```python
from build123d import *

# Parameters (mm, degrees)
SKETCH_1_R          = 26
SKETCH_1_R_2        = 24
EXTRUDE_1_DEPTH     = 12.6
EXTRUDE_START       = -2
SKETCH_2_R          = 28
SKETCH_2_R_2        = 26
EXTRUDE_2_DEPTH     = 2
SKETCH_3_R          = 26
EXTRUDE_3_DEPTH     = 2
SKETCH_4_R          = 26
SKETCH_4_R_2        = 22
EXTRUDE_4_DEPTH     = 1
EXTRUDE_START_2     = 11
EXTRUDE_5_DEPTH     = 11
M3X0_51_D           = 2.5
SKETCH_8_R          = 7
CUT_EXTRUDE_1_DEPTH = 2
HOLE_WIZARD_M31_D   = 3.4


with BuildPart() as part:
    # Эскиз1 → Бобышка-Вытянуть1 (new body)
    with BuildSketch(Plane(origin=(0, 0, 0), x_dir=(1, 0, 0), z_dir=(0, 1, 0))):
        with Locations(Location((0, 0, 0), (0, 0, 270))):
            Circle(SKETCH_1_R)
        with Locations(Location((0, 0, 0), (0, 0, 270))):
            Circle(SKETCH_1_R_2, mode=Mode.SUBTRACT)
    extrude(amount=EXTRUDE_1_DEPTH)

    # Эскиз2 → Бобышка-Вытянуть2 (add)
    with BuildSketch(Plane.XZ.offset(EXTRUDE_START)):
        with Locations(Location((0, 0, 0), (0, 0, 270))):
            Circle(SKETCH_2_R)
        with Locations(Location((0, 0, 0), (0, 0, 270))):
            Circle(SKETCH_2_R_2, mode=Mode.SUBTRACT)
    extrude(amount=EXTRUDE_2_DEPTH)

    # Эскиз3 → Бобышка-Вытянуть3 (add)
    with BuildSketch(Plane(origin=(0, 12.6, 0), x_dir=(1, 0, 0), z_dir=(0, 1, 0))):
        with Locations(Location((0, 0, 0), (0, 0, 90))):
            Circle(SKETCH_3_R)
    extrude(amount=EXTRUDE_3_DEPTH)

    # Эскиз4 → Бобышка-Вытянуть4 (add)
    with BuildSketch(Plane(origin=(0, 14.6, 0), x_dir=(1, 0, 0), z_dir=(0, 1, 0))):
        with Locations(Location((0, 0, 0), (0, 0, 90))):
            Circle(SKETCH_4_R)
        with Locations(Location((0, 0, 0), (0, 0, 270))):
            Circle(SKETCH_4_R_2, mode=Mode.SUBTRACT)
    extrude(amount=EXTRUDE_4_DEPTH)

    # Эскиз5 → Бобышка-Вытянуть5 (add)
    with BuildSketch(Plane.XZ.offset(-12.6).offset(EXTRUDE_START_2)):
        with BuildLine():
            Line((19, 3.5), (23.743420141, 3.5))
            ThreePointArc((23.743420141, 3.5), (24, 0), (23.743420141, -3.5))
            Line((23.743420141, -3.5), (19, -3.5))
            ThreePointArc((19, -3.5), (15.5, 0), (19, 3.5))
        make_face()
        with BuildLine():
            Line((-19, -3.5), (-23.743420141, -3.5))
            ThreePointArc((-23.743420141, -3.5), (-24, 0), (-23.743420141, 3.5))
            Line((-23.743420141, 3.5), (-19, 3.5))
            ThreePointArc((-19, 3.5), (-15.5, 0), (-19, -3.5))
        make_face()
    extrude(amount=-EXTRUDE_5_DEPTH)

    # Отверстие обработанное метчиком M3x0.51 (through all)
    with Locations(Plane(origin=(0, 1.6, 0), x_dir=(-1, 0, 0), z_dir=(0, -1, 0))):
        with Locations((-19, 0), (19, 0)):
            Hole(M3X0_51_D / 2)

    # Эскиз8 → Вырез-Вытянуть1 (cut)
    with BuildSketch(Plane(origin=(0, 14.6, 0), x_dir=(1, 0, 0), z_dir=(0, 1, 0))):
        with Locations(Location((0, 0, 0), (0, 0, 270))):
            Circle(SKETCH_8_R)
    extrude(amount=-CUT_EXTRUDE_1_DEPTH, mode=Mode.SUBTRACT)

    # Отверстие с зазором M31 (through all)
    with Locations(Plane(origin=(0, 14.6, 0), x_dir=(1, 0, 0), z_dir=(0, 1, 0))):
        with Locations((-8.838834765, 8.838834765), (8.838834765, 8.838834765), (8.838834765, -8.838834765), (-8.838834765, -8.838834765)):
            Hole(HOLE_WIZARD_M31_D / 2)


solid = part.part
```
Geometry: final body of the model. Coordinates: model frame, mm. A direction names the side the tool comes from. Round coordinates to 2 decimals unless told otherwise and drop trailing zeros. Order: outer loops, then holes, each group sorted by start corner. A loop starts at its lowest first (then second) coordinate and runs counter-clockwise, first axis right, second up. Notation, with made-up numbers: (27, -4) -> (53, -4) arc R15 cw to (53, 14) -> close; hole circle Ø4 at (59.25, 89.5). An arc over 180 degrees is marked (long way). Use CSV: the item, a comma, the result in double quotes. Start each with the question number.
1) Material intervals for line 1 along Z through (x, y) = (-20, 9); line 2 along Z through (x, y) = (-19, 6.25); line 3 along X through (y, z) = (15.05, 0), sorted ascending. Write a range as from..to.
2) Draft query along Z for faces 1 (the face through (13, 0, -21)), 2 (the face through (-27.334, 1.014, 6.07)), 3 (the face through (20.155, 8.191, 0.479)). Return one class per face: +Z half, -Z half, draft (parallel to the pull), parting line (faces both ways), or undercut.
3) Section C-C (y = 4.5). Return the cut outline in (x, z), and give its area (3 significant figures).
4) First-contact query: pin 1 Ø2.5 at (x, y) = (21, 5) entering from +Z; pin 2 Ø2 at (x, y) = (-11, 9.5) entering from +Z; pin 3 Ø4 at (x, z) = (-12, -14.5) entering from +Y; pin 4 Ø3 at (x, z) = (-8.84, 8.84) entering from -Y. Flat tips, straight axial feed; report the tip coordinate or a pass-through.
5) Section A-A (x = 0). Return the cut outline in (y, z).
6) Section D-D (z = 8). Return the cut outline in (x, y), and give its area (3 significant figures).
7) Section B-B (z = 0). State how many separate pieces and enclosed holes the cut face has, and give its area (3 significant figures).
8) Set-up query: faces 4 (the face through (9.21, 13.59, -7.18)), 5 (the face through (-5.2, 14.6, 5.2)), 6 (the face through (5, 12.6, 6)). Return all of +Z, -Z, +X, -X, +Y, -Y with unobstructed straight access to the full face (end or side cutting, diameter ignored); none if empty.
Returned:
1,line 1,"z = -16.61..-13.27, -3.5..-0.75, 0.75..3.5, 13.27..16.61"
1,line 2,"z = -17.75..-14.66, -3.5..-1.25, 1.25..3.5, 14.66..17.75"
1,line 3,"x = -26..-22, 22..26"
2,face 1,"draft"
2,face 2,"parting line"
2,face 3,"undercut"
3,outline,"circle Ø52 at (0, 0); hole (-23.74, -3.5) arc R24 ccw to (23.74, -3.5) -> (19, -3.5) arc R3.5 cw to (19, 3.5) -> (23.74, 3.5) arc R24 ccw to (-23.74, 3.5) -> (-19, 3.5) arc R3.5 cw to (-19, -3.5) -> close; hole circle Ø2.5 at (-19, 0); hole circle Ø2.5 at (19, 0)"
3,area,"412 mm²"
4,pin 1,"stops at z = 16.91"
4,pin 2,"stops at z = 24"
4,pin 3,"stops at y = 14.6"
4,pin 4,"passes through"
5,outline,"(0, -28) -> (2, -28) -> (2, -26) -> (15.6, -26) -> (15.6, -22) -> (14.6, -22) -> (14.6, -7) -> (12.6, -7) -> (12.6, -24) -> (0, -24) -> close; (0, 24) -> (12.6, 24) -> (12.6, 7) -> (14.6, 7) -> (14.6, 22) -> (15.6, 22) -> (15.6, 26) -> (2, 26) -> (2, 28) -> (0, 28) -> close"
6,outline,"(-26.83, 0) -> (-22.63, 0) -> (-22.63, 12.6) -> (-10.32, 12.6) -> (-10.32, 14.6) -> (-20.49, 14.6) -> (-20.49, 15.6) -> (-24.74, 15.6) -> (-24.74, 2) -> (-26.83, 2) -> close; (-7.36, 12.6) -> (7.36, 12.6) -> (7.36, 14.6) -> (-7.36, 14.6) -> close; (10.32, 12.6) -> (22.63, 12.6) -> (22.63, 0) -> (26.83, 0) -> (26.83, 2) -> (24.74, 2) -> (24.74, 15.6) -> (20.49, 15.6) -> (20.49, 14.6) -> (10.32, 14.6) -> close"
6,area,"157 mm²"
7,separate pieces,"4"
7,enclosed holes,"0"
7,area,"264 mm²"
8,face 4,"+Y, -Y"
8,face 5,"+Y"
8,face 6,"-Y"
